Autodesk Inventor part; units mm, degrees
ref_plane "YZ Plane" through (0, 0, 0) normal (1, 0, 0) x (0, 1, 0)
ref_plane "XZ Plane" through (0, 0, 0) normal (0, 1, 0) x (-1, 0, 0)
ref_plane "XY Plane" through (0, 0, 0) normal (0, 0, 1) x (1, 0, 0)
sketch "Szkic1" plane through (0, 0, 0) normal (1, 0, 0) x (0, 1, 0)
  line L0 (10, 10) -> (-10, 10)
  line L1 (-10, 10) -> (-10, -10)
  line L2 (-10, -10) -> (10, -10)
  line L3 (10, -10) -> (10, 10)
  line L4 (0, 0) -> (10, 0) construction
  line L5 (0, 0) -> (0, -10) construction
  dimension "d0" = 20
  dimension "d1" = 20
extrude "Wyciągnięcie proste1" add sketch "Szkic1" along normal blind 10
sketch "Szkic2" plane through (10, 0, 0) normal (1, 0, 0) x (0, 0, -1)
  line L0 (10, -10) -> (10, 10)
  point P0 (0, 0)
  point P1 (4, 0)
  dimension "d4" = 6
hole "Otwór1" at (10, 0, -4) direction (-1, 0, 0) diameter 6 end through all
sketch "Szkic3" plane through (0, -10, -10) normal (0, -1, 0) x (1, 0, 0)
  line L0 (0, 20) -> (0, 0)
  line L1 (0, 20) -> (10, 20)
  point P0 (0, 10)
  point P1 (5, 15)
  dimension "d12" = 5
  dimension "d13" = 5
hole "Otwór2" at (5, -10, 5) direction (0, 1, 0) diameter 6 end through all
sketch "Szkic4" plane through (0, -10, -10) normal (0, -1, 0) x (1, 0, 0)
  line L0 (0, 20) -> (0, 0)
  point P0 (0, 10)
  point P1 (3, 10)
  point P2 (0, 10)
  dimension "d21" = 3
hole "Otwór3" at (3, -10, 0) direction (0, 1, 0) diameter 2 depth 5 tip angle 118
sketch "Szkic5" plane through (10, 0, 0) normal (1, 0, 0) x (0, 0, -1)
  line L0 (-2, -10) -> (-8, -10)
  line L1 (-10, 10) -> (-10, -10)
  point P0 (0, 0)
  point P1 (-5, 0)
  dimension "d29" = 5
hole "Otwór4" at (10, 0, 5) direction (-1, 0, 0) diameter 3 depth 5 tip angle 118
thread "Gwint1"
thread "Gwint2"
fillet "Zaokrąglenie1" radius 0.5 12 edges at (0, 0, 10) (0, -10, 0) (5, -10, 10) (10, -10, 0) (10, 0, 10) (5, -10, -10) (0, 0, -10) (10, 0, -10) (5, 10, -10) (0, 10, 0) (10, 10, 0) (5, 10, 10)
properties part number "HotBlock"
Model file for the job. Use its own axes, mm. A direction names the side the tool comes from. Give positions to 0.01 mm unless a question says otherwise; leave off trailing zeros. Loops run counter-clockwise (first coordinate to the right, second up) from the corner with the lowest first, then second, coordinate; pieces in that order, holes last.
1) Wall check: line 1 (Z direction, x = 8.45, y = 0); line 2 (X direction, y = -5.25, z = 0); line 3 (Y direction, x = 9.05, z = 5). Give the ranges that are in metal, low to high.
2) Tool access for faces 4 (the cylindrical face through (2, 0, 5)), 5 (the cylindrical face through (4, -7, 0)): list every direction of +Z, -Z, +X, -X, +Y, -Y with a clear straight run to the whole face (end or side of a thin tool).
3) Saw through at B-B (y = -5.75). Write the cut outline in (x, z), plus the area to 3 significant figures.
4) Pull direction Y, two halves, no side cores. Call faces 1 (the cylindrical face through (8.782, 0.575, 3.614)), 2 (the flat face through (5, 0, -10)), 3 (the flat face through (5, -10, 0)): +Y half, -Y half, draft (parallel to the pull), parting line (faces both ways), or undercut.
5) Saw through at D-D (y = 1.75). Write the cut outline in (x, z).
6) Saw through at C-C (z = 5). Write the cut outline in (x, y).
7) Saw through at A-A (x = 5). Write the cut outline in (y, z), plus the area to 3 significant figures.
Answer block:
1. line 1: z = -10 to -7, -1 to 3.5, 6.5 to 10
1. line 2: x = 0 to 2, 4 to 10
1. line 3: y = -10 to -1.5, 1.5 to 10
2. face 4: +Y, -Y
2. face 5: -Y
3. outline: (0, -9.5) arc R0.5 ccw to (0.5, -10) - (9.5, -10) arc R0.5 ccw to (10, -9.5) - (10, 9.5) arc R0.5 ccw to (9.5, 10) - (0.5, 10) arc R0.5 ccw to (0, 9.5) - close; hole circle Ø2 at (3, 0); hole circle Ø6 at (5, 5)
3. area: 168 mm2
4. face 1: undercut
4. face 2: draft
4. face 3: -Y half
5. outline: (0, -9.5) arc R0.5 ccw to (0.5, -10) - (9.5, -10) arc R0.5 ccw to (10, -9.5) - (10, -6.44) - (0, -6.44) - close; (0, -1.56) - (10, -1.56) - (10, 9.5) arc R0.5 ccw to (9.5, 10) - (0.5, 10) arc R0.5 ccw to (0, 9.5) - close; hole circle Ø6 at (5, 5)
6. outline: (0, -9.5) arc R0.5 ccw to (0.5, -10) - (2, -10) - (2, 10) - (0.5, 10) arc R0.5 ccw to (0, 9.5) - close; (8, -10) - (9.5, -10) arc R0.5 ccw to (10, -9.5) - (10, -1.5) - (8, -1.5) - close; (8, 1.5) - (10, 1.5) - (10, 9.5) arc R0.5 ccw to (9.5, 10) - (8, 10) - close
7. outline: (-10, -9.5) arc R0.5 ccw to (-9.5, -10) - (9.5, -10) arc R0.5 ccw to (10, -9.5) - (10, 2) - (-10, 2) - close; (-10, 8) - (10, 8) - (10, 9.5) arc R0.5 ccw to (9.5, 10) - (-9.5, 10) arc R0.5 ccw to (-10, 9.5) - close; hole circle Ø6 at (0, -4)
7. area: 252 mm2
